The model under review builds one solid part; all positions refer to its coordinate system, in mm. A direction names the side the tool comes from. Round coordinates to 2 decimals unless told otherwise and drop trailing zeros. Order: outer loops, then holes, each group sorted by start corner. A loop starts at its lowest first (then second) coordinate and runs counter-clockwise, first axis right, second up.
from build123d import *

# Parameters (mm, degrees)
BOSS_EXTRUDE1_DEPTH = 53.99999995
HOLE1_D             = 6.99999997
HOLE2_D             = 30.999999976
HOLE2_CBORE_D       = 40.00000001
HOLE2_CBORE_DEPTH   = 11.999999876


with BuildPart() as part:
    # Sketch1 → Boss-Extrude1 (new body)
    with BuildSketch(Plane.XY):
        Polygon((-21.999999942, 56.999999919), (-14.999999972, 56.999999919), (-14.999999972, 26.999999975), (14.999999972, 26.999999975), (14.999999972, 56.999999919), (21.999999942, 56.999999919), (21.999999942, -56.999999919), (14.999999972, -56.999999919), (14.999999972, -26.999999975), (-14.999999972, -26.999999975), (-14.999999972, -56.999999919), (-21.999999942, -56.999999919), align=None)
    extrude(amount=BOSS_EXTRUDE1_DEPTH)

    # Hole1 (through all)
    with Locations(Plane.ZY.offset(21.999999942)):
        with Locations((26.999999975, 41.999999947), (26.999999975, -41.999999947)):
            Hole(HOLE1_D / 2)

    # Hole2 (through all)
    with Locations(Plane.ZY.offset(21.999999942)):
        with Locations((26.999999975, 0)):
            CounterBoreHole(HOLE2_D / 2, HOLE2_CBORE_D / 2, HOLE2_CBORE_DEPTH)


solid = part.part
(1) Tool access review of faces 1 (the flat face through (0, 27, 27)), 2 (the cylindrical face through (-16.084, 6.007, 46.076)), 3 (the flat face through (19, -57, 27)): name each direction out of +Z, -Z, +X, -X, +Y, -Y from which nothing blocks a thin tool from reaching the whole face with its end or side.
(2) We need section C-C (x = 10). Give the boundary of the cut face in (y, z).
(3) Clearance check with flat-ended pins moving along their axes: P1, Ø12, axis at x = 4.5, z = 30.5, coming from the +Y side; P2, Ø1.5, axis at x = -0.5, z = 31, coming from the -Y side; P3, Ø24, axis at y = 0, z = 27, coming from the +X side. State where each tip first meets the part, or that it passes through.
(4) The part is to be moulded in two halves that separate along Y. For faces 4 (the flat face through (0, -27, 27)), 5 (the flat face through (15, -46, 27)), 6 (the cylindrical face through (-18.451, -39.635, 29.58)), say which applies: pulls with the +Y half, pulls with the -Y half, needs draft (parallel to the pull), parting line crosses it, or undercut.
(5) We need section B-B (z = 32.5). Give the boundary of the cut face in (x, y), and give its area (3 significant figures).
(6) We need section A-A (y = -42). Give the boundary of the cut face in (x, z), and give its area (3 significant figures).
(7) We need section D-D (y = 0). Give the boundary of the cut face in (x, z), and give its area (3 significant figures).
(8) To check wall thickness, follow L1, parallel to Y at x = -18, z = 27; L2, parallel to Y at x = 19.75, z = 27; L3, parallel to Z at x = -17, y = 42. State the ranges of each line that lie inside material, in increasing order.
Verdict:
1. face 1: +Z, -Z, +Y
1. face 2: -X
1. face 3: +Z, -Z, +X, -X, -Y
2. outline: (-27, 0) - (27, 0) - (27, 54) - (-27, 54) - close; hole circle Ø31 at (0, 27)
3. P1: stops at y = 27
3. P2: stops at y = -27
3. P3: passes through
4. face 4: pulls with the -Y half
4. face 5: needs draft
4. face 6: undercut
5. outline: (-22, -57) - (-15, -57) - (-15, -27) - (15, -27) - (15, -57) - (22, -57) - (22, -14.49) - (-10, -14.49) - (-10, -19.23) - (-22, -19.23) - close; (-22, 19.23) - (-10, 19.23) - (-10, 14.49) - (22, 14.49) - (22, 57) - (15, 57) - (15, 27) - (-15, 27) - (-15, 57) - (-22, 57) - close
5. area: 1,830 mm2
6. outline: (-22, 0) - (-15, 0) - (-15, 23.5) - (-22, 23.5) - close; (-22, 30.5) - (-15, 30.5) - (-15, 54) - (-22, 54) - close; (15, 0) - (22, 0) - (22, 23.5) - (15, 23.5) - close; (15, 30.5) - (22, 30.5) - (22, 54) - (15, 54) - close
6. area: 658 mm2
7. outline: (-22, 0) - (22, 0) - (22, 11.5) - (-10, 11.5) - (-10, 7) - (-22, 7) - close; (-22, 47) - (-10, 47) - (-10, 42.5) - (22, 42.5) - (22, 54) - (-22, 54) - close
7. area: 904 mm2
8. L1: y = -57 to -45.5, -38.5 to -20, 20 to 38.5, 45.5 to 57
8. L2: y = -57 to -45.5, -38.5 to -15.5, 15.5 to 38.5, 45.5 to 57
8. L3: z = 0 to 23.5, 30.5 to 54
